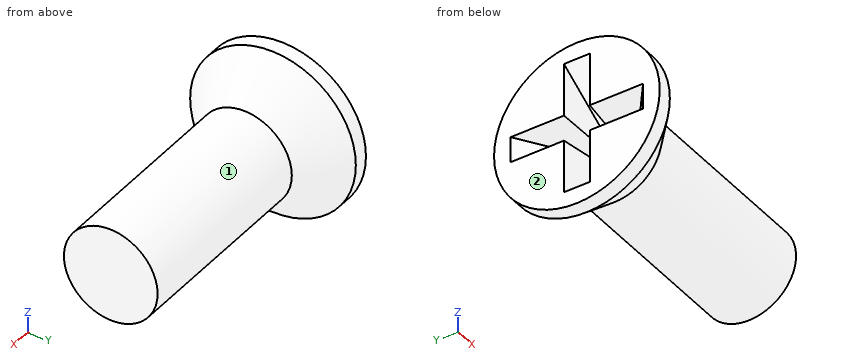
```python
from build123d import *

# Parameters (mm, degrees)
SKETCH3_W         = 0.9652
SKETCH3_H         = 4.953
SKETCH4_W         = 0.4826
SKETCH4_H         = 0.4826
CIRPATTERN1_COUNT = 2
CIRPATTERN1_ANGLE = 90


with BuildPart() as part:
    # BodySke → Base-Revolve (revolve)
    with BuildSketch(Plane.XY):
        Polygon((0, 0), (0, 3.0988), (0.55957405, 3.0988), (2.1082, 1.7526), (9.525, 1.7526), (9.525, 0), align=None)
    revolve(axis=Axis((-6.35, 0, 0), (1, 0, 0)))

    # Sketch3 → Cross section 0
    with BuildSketch(Plane.ZY):
        Rectangle(SKETCH3_W, SKETCH3_H)
    # Sketch4 → Cross section 1
    with BuildSketch(Plane.ZY.offset(-2.8702)):
        Rectangle(SKETCH4_W, SKETCH4_H)
    cross = loft(mode=Mode.SUBTRACT)

    # CirPattern1: Cross ×2 about axis
    cirpattern1_axis = Axis((0, 0, 0), (1, 0, 0))
    for i in range(1, CIRPATTERN1_COUNT):
        add(cross.rotate(cirpattern1_axis, i * CIRPATTERN1_ANGLE / (CIRPATTERN1_COUNT - 1)), mode=Mode.SUBTRACT)


solid = part.part
```
Build history of the part. All positions in model axes, mm. Face numbers are marked on the shaded views. A direction names the side the tool comes from. Round coordinates to 2 decimals unless told otherwise and drop trailing zeros. Write each loop counter-clockwise with the first axis right and the second up, starting at its lowest first coordinate (ties: lowest second). Pieces come first, ordered by that corner, then holes. Notation, with made-up numbers: (-9, -29) -> (-1, -29) arc R25 cw to (-1, -13) -> close; hole circle Ø9 at (-28.5, -10.5). An arc over 180 degrees is marked (long way). Put each result on its own line as item: value.
Item 1: Slice it at A-A, the plane x = 5.5. Give the cut face in (y, z), plus the area to 3 significant figures.
Here are the results:
outline: circle Ø3.51 at (0, 0)
area: 9.65 mm^2
Item 2: Wall check: probe 1 along Y at (x, z) = (1.25, -0.25); probe 2 along Z at (x, y) = (5.25, 0.5); probe 3 along Y at (x, z) = (2.25, -0.5). Give the ranges that are in metal, low to high. Write a range as from..to.
Here are the results:
probe 1: y = -2.49..-1.5, 1.5..2.49
probe 2: z = -1.68..1.68
probe 3: y = -1.68..-0.29, 0.29..1.68
Item 3: Tool access for the marked faces 1 and 2: list every direction of +Z, -Z, +X, -X, +Y, -Y with a clear straight run to the whole face (end or side of a thin tool).
Here are the results:
face 1: +X
face 2: +Z, -Z, -X, +Y, -Y
